Design review of the part built by this model. Coordinates are the model's own, in mm. Give positions to 0.01 mm unless a question says otherwise; leave off trailing zeros. Write each loop counter-clockwise with the first axis right and the second up, starting at its lowest first coordinate (ties: lowest second). Pieces come first, ordered by that corner, then holes. Notation, with made-up numbers: (71, -4) - (116, -4) arc R23 cw to (116, 8) - close; hole circle Ø5 at (-12.75, 64). An arc over 180 degrees is marked (long way). Use a Markdown table: item, result. Add a question column.
```python
from build123d import *

# Parameters (mm, degrees)
F0_W     = 101.6
F0_H     = 101.6
F0_R     = 12.7
F1_DEPTH = 25.4


with BuildPart() as f1:
    # F0 (on Front) → F1 (new body)
    with BuildSketch(Plane.XZ):
        with Locations((3.532663, 3.283243)):
            Rectangle(F0_W, F0_H)
        with Locations((-30.266313, -32.366816)):
            Circle(F0_R, mode=Mode.SUBTRACT)
        with Locations((0, -32.557767)):
            Circle(F0_R, mode=Mode.SUBTRACT)
        Circle(F0_R, mode=Mode.SUBTRACT)
        with Locations((40.577866, -31.412043)):
            Circle(F0_R, mode=Mode.SUBTRACT)
        with Locations((40.386911, 0)):
            Circle(F0_R, mode=Mode.SUBTRACT)
        with Locations((-31.412043, 3.283243)):
            Circle(F0_R, mode=Mode.SUBTRACT)
        with Locations((-32.939676, 37.713546)):
            Circle(F0_R, mode=Mode.SUBTRACT)
        with Locations((0, 37.331637)):
            Circle(F0_R, mode=Mode.SUBTRACT)
        with Locations((40.959772, 38.095452)):
            Circle(F0_R, mode=Mode.SUBTRACT)
    extrude(amount=F1_DEPTH)


solid = f1.part
```
(1) Add section B-B (z = 34). State the section outline as (x, y) points, and give its area (3 significant figures).
(2) Mouldability with a two-part tool opening along X and no side actions: class faces 1 (the face through (3, -13, 54.083)), 2 (the face through (-47.267, -13, 3)), 3 (the face through (-1.653, -12.522, 49.924)), 4 (the face through (54.333, -13, 3)) as +X half, -X half, draft (parallel to the pull), parting line (faces both ways), or undercut.
(3) For line 1 along Z through (x, y) = (0, -12); line 2 along X through (y, z) = (-18.25, -26); line 3 along Z through (x, y) = (49, -21.5), list the stretches that pass through material, from the lowest coordinate up.
(4) Add section C-C (y = -9.5). Count the separate pieces of the cut face and the enclosed holes in it, and give its area (3 significant figures).
(5) Add section A-A (x = 0). State the section outline as (y, z) points, and give its area (3 significant figures).
Answers follow:
| question | item | result |
|---|---|---|
| 1 | outline | (-47.27, -25.4) - (-45.08, -25.4) - (-45.08, 0) - (-47.27, 0) - close; (-20.79, -25.4) - (-12.26, -25.4) - (-12.26, 0) - (-20.79, 0) - close; (12.26, -25.4) - (28.94, -25.4) - (28.94, 0) - (12.26, 0) - close; (52.98, -25.4) - (54.33, -25.4) - (54.33, 0) - (52.98, 0) - close |
| 1 | area | 730 mm^2 |
| 2 | face 1 | draft |
| 2 | face 2 | -X half |
| 2 | face 3 | undercut |
| 2 | face 4 | +X half |
| 3 | line 1 | -47.52 to -45.26, -19.86 to -12.7, 12.7 to 24.63, 50.03 to 54.08 |
| 3 | line 2 | -47.27 to -41.26, -19.28 to -10.88, 10.88 to 29.09, 52.07 to 54.33 |
| 3 | line 3 | -47.52 to -40.92, -21.91 to -9.33, 9.33 to 28.26, 47.93 to 54.08 |
| 4 | separate pieces | 1 |
| 4 | enclosed holes | 9 |
| 4 | area | 5,760 mm^2 |
| 5 | outline | (-25.4, -47.52) - (0, -47.52) - (0, -45.26) - (-25.4, -45.26) - close; (-25.4, -19.86) - (0, -19.86) - (0, -12.7) - (-25.4, -12.7) - close; (-25.4, 12.7) - (0, 12.7) - (0, 24.63) - (-25.4, 24.63) - close; (-25.4, 50.03) - (0, 50.03) - (0, 54.08) - (-25.4, 54.08) - close |
| 5 | area | 645 mm^2 |
